Here's how the part is built. I have some questions about the finished solid (model axes, mm). Face numbers are marked on the shaded views. A direction names the side the tool comes from. Round coordinates to 2 decimals unless told otherwise and drop trailing zeros. Loops run counter-clockwise (first coordinate to the right, second up) from the corner with the lowest first, then second, coordinate; pieces in that order, holes last. Notation, with made-up numbers: M -4.75,-26.75 L 10.25,-26.75 A18 ccw 10.25,-18.75 Z; hole C -15,-9 d6. An arc over 180 degrees is marked long. Write each question's results on one line, items separated by ' | '. Start each with the question number.
Autodesk Inventor part; units mm, degrees
ref_plane "YZ Plane" through (0, 0, 0) normal (1, 0, 0) x (0, 1, 0)
ref_plane "XZ Plane" through (0, 0, 0) normal (0, 1, 0) x (-1, 0, 0)
ref_plane "XY Plane" through (0, 0, 0) normal (0, 0, 1) x (1, 0, 0)
sketch "Sketch1" plane through (0, 0, 0) normal (0, 1, 0) x (-1, 0, 0)
  line L0 (1, -18.473) -> (1, -4.6435)
  line L1 (1, 4.6435) -> (1, 18.473)
  line L2 (-1, -18.473) -> (-1, -4.6435)
  line L3 (-1, 4.6435) -> (-1, 18.473)
  line L4 (18.473, 1) -> (4.6435, 1)
  line L5 (-4.6435, 1) -> (-18.473, 1)
  line L6 (18.473, -1) -> (4.6435, -1)
  line L7 (-4.6435, -1) -> (-18.473, -1)
  arc A0 (-18.473, 1) -> (-18.473, -1) centre (0, 0) ccw
  arc A1 (-1, -18.473) -> (1, -18.473) centre (0, 0) ccw
  arc A2 (18.473, -1) -> (18.473, 1) centre (0, 0) ccw
  arc A3 (1, 18.473) -> (-1, 18.473) centre (0, 0) ccw
  arc A4 (4.6435, 1) -> (1, 4.6435) centre (0, 0) ccw
  arc A5 (-1, 4.6435) -> (-4.6435, 1) centre (0, 0) ccw
  arc A6 (-4.6435, -1) -> (-1, -4.6435) centre (0, 0) ccw
  arc A7 (1, -4.6435) -> (4.6435, -1) centre (0, 0) ccw
  point P0 (1, -4.899)
  point P1 (1, 4.899)
  point P2 (4.899, -1)
  point P3 (-1, 4.899)
  point P4 (4.899, 1)
  point P5 (-4.899, 1)
  point P6 (-4.899, -1)
  point P7 (-1, -4.899)
  point P8 (-18.9737, -1)
  point P9 (-1, -18.9737)
  point P10 (1, -18.9737)
  point P11 (18.9737, -1)
  point P12 (18.9737, 1)
  point P13 (1, 18.9737)
  point P14 (-1, 18.9737)
  point P15 (-18.9737, 1)
  point P16 (17.4714, 1)
  point P17 (1, 17.4714)
  point P18 (-1, 17.4714)
  point P19 (-17.4714, 1)
  point P20 (-17.4714, -1)
  point P21 (-1, -17.4714)
  point P22 (1, -17.4714)
  point P23 (17.4714, -1)
extrude "Extrusion1" add sketch "Sketch1" along normal blind 9
sketch "Sketch2" plane through (0, 0, 0) normal (0, -1, 0) x (1, 0, 0)
  circle A0 centre (0, 0) radius 4.75
  dimension "d11" = 9.5
extrude "Extrusion2" add sketch "Sketch2" along normal blind 2
sketch "Sketch3" plane through (0, 9, 0) normal (0, 1, 0) x (1, 0, 0)
  arc A0 (2.75, 0) -> (0, -2.75) centre (0, 0) ccw
  line L0 (0, -2.75) -> (2.75, 0)
  dimension "d6" = 5.5
extrude "Extrusion3" cut sketch "Sketch3" against normal through all
properties part number "wheel of the walls"
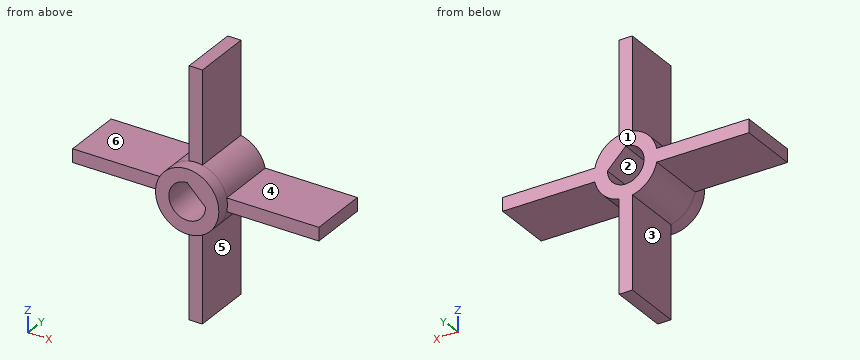
1. I want a section at A-A on y = 6.75. List the corners of the cut face in (x, z) for me, plus the area to 3 significant figures.
2. Which directions (+Z, -Z, +X, -X, +Y, -Y) give clear straight access to the entire face, cutting with the end or side of a thin tool? Please do the marked faces 4, 5 and 6.
3. For pin 1 (0.6 mm diameter, centred on x = 0.5, z = 14.5, fed in from -Y); pin 2 (1.5 mm diameter, centred on x = -3, y = 2, fed in from +Z); pin 3 (5 mm diameter, centred on x = 8, z = -4.5, fed in from -Y); pin 4 (2.5 mm diameter, centred on x = 12.5, y = 5.5, fed in from -Z), each with a flat end and sliding along its axis, tell me the tip position at first contact or that it passes through.
4. I want a section at C-C on x = -14. List the corners of the cut face in (y, z) for me, plus the area to 3 significant figures.
5. I want a section at D-D on z = -9.5. List the corners of the cut face in (x, y) for me, plus the area to 3 significant figures.
6. If we mould it in two halves opening along X, with no side actions, what happens to the marked faces 1, 2 and 3? For each: released by +X, released by -X, zero draft, split by the parting line, or undercut.
7. I want a section at B-B on z = 0.5. List the corners of the cut face in (x, y) for me.
8. I need wall thicknesses on line 1 along X through (y, z) = (0.75, -6); line 2 along Y through (x, z) = (13, 0). Which ranges of each line are inside material? Lowest first, please.
Outcome:
1) outline: M -18.47,-1 L -4.64,-1 A4.75 ccw -1,-4.64 L -1,-18.47 A18.5 ccw 1,-18.47 L 1,-4.64 A4.75 ccw 4.64,-1 L 18.47,-1 A18.5 ccw 18.47,1 L 4.64,1 A4.75 ccw 1,4.64 L 1,18.47 A18.5 ccw -1,18.47 L -1,4.64 A4.75 ccw -4.64,1 L -18.47,1 A18.5 ccw Z; hole M 0,2.75 A2.75 ccw long 2.75,0 Z | area: 159 mm2
2) face 4: +Z, +X, +Y, -Y | face 5: -Z, +X, +Y, -Y | face 6: +Z, -X, +Y, -Y
3) pin 1: y = 0 | pin 2: z = 4.18 | pin 3: through | pin 4: z = -1
4) outline: M 0,-1 L 9,-1 L 9,1 L 0,1 Z | area: 18.0 mm2
5) outline: M -1,0 L 1,0 L 1,9 L -1,9 Z | area: 18.0 mm2
6) face 1: zero draft | face 2: undercut | face 3: released by -X
7) outline: M -18.49,0 L -4.72,0 L -4.72,-2 L -2.7,-2 L -2.7,9 L -18.49,9 Z; M 2.25,-2 L 4.72,-2 L 4.72,0 L 18.49,0 L 18.49,9 L 2.25,9 Z
8) line 1: -1 to 1 | line 2: 0 to 9
